```python
from build123d import *

# Parameters (mm, degrees)
F1_DEPTH = 63.5
F0_W     = 22.4716843884
F0_H     = 19.05
F2_DEPTH = 25.4
F3_DEPTH = 15.875
F5_R     = 6.35


# Not quite as in the source:
# - the program builds the solid bodies; features that only make, move or delete a surface that nothing else refers to are left out


with BuildPart() as f1:
    # F0 (on Front) → F1 (new body, symmetric)
    with BuildSketch(Plane.XZ):
        Polygon((22.225, 9.525), (-41.275, 9.525), (-41.275, -9.525), (41.275, -9.525), (41.275, 9.525), align=None)
    extrude(amount=F1_DEPTH, both=True)

    # F0 (on Front) → F2 (join, symmetric)
    with BuildSketch(Plane.XZ):
        with BuildLine():
            Line((22.225, 27.0002), (22.225, 9.525))
            Line((22.225, 9.525), (41.275, 9.525))
            Line((41.275, 9.525), (41.275, 27.0002))
            ThreePointArc((41.275, 27.0002), (45.9246798487, 38.2255201513), (57.15, 42.8752))
            Line((57.15, 42.8752), (60.325, 42.8752))
            Line((60.325, 42.8752), (60.325, 61.9252))
            Line((60.325, 61.9252), (57.15, 61.9252))
            ThreePointArc((57.15, 61.9252), (32.4542956671, 51.6959043329), (22.225, 27.0002))
        make_face()
        with Locations((71.5608421942, 52.4002)):
            Rectangle(F0_W, F0_H)
    extrude(amount=F2_DEPTH, both=True)

    # F0 (on Front) → F3 (join)
    with BuildSketch(Plane.XZ):
        with BuildLine():
            add(Edge.make_bspline(
                [(-41.275, 9.525), (-37.7052687109, 41.8739132583), (35.1902469993, 68.9807906747), (57.15, 61.9252)],
                knots=[0, 0, 0, 0, 111.5045361635, 111.5045361635, 111.5045361635, 111.5045361635], degree=3))
            Line((-41.275, 9.525), (22.225, 9.525))
            Line((22.225, 9.525), (22.225, 27.0002))
            ThreePointArc((22.225, 27.0002), (32.4542956671, 51.6959043329), (57.15, 61.9252))
        make_face()
    extrude(amount=F3_DEPTH)

    # F5
    f5_edges = [f1.edges().sort_by_distance(p)[0] for p in [
        (41.275, -63.5, 0),
        (-41.275, -63.5, 0),
        (-41.275, 63.5, 0),
        (41.275, 63.5, 0),
    ]]
    fillet(f5_edges, radius=F5_R)


solid = f1.part
```
Read the model definition and answer for the solid it produces. Units are mm, in the model's axes. A direction names the side the tool comes from. Round coordinates to 2 decimals unless told otherwise and drop trailing zeros. Write each loop counter-clockwise with the first axis right and the second up, starting at its lowest first coordinate (ties: lowest second). Pieces come first, ordered by that corner, then holes. Notation, with made-up numbers: (11.5, -29.75) - (53.5, -29.75) arc R18 cw to (53.5, -23.75) - close; hole circle Ø4 at (48, 53.5). An arc over 180 degrees is marked (long way). One line per item, written item: value.
Q1. Find section D-D (y = 35.5). Determine the outline of the cut face in (x, z) (3 decimals), and give its area (3 significant figures).
The answers:
outline: (-41.275, -9.525) - (41.275, -9.525) - (41.275, 9.525) - (-41.275, 9.525) - close
area: 1,570 mm2
Q2. Find section A-A (z = 2.5). Determine the outline of the cut face in (x, y) (3 decimals), and give its area (3 significant figures).
The answers:
outline: (-41.275, -57.15) arc R6.35 ccw to (-34.925, -63.5) - (34.925, -63.5) arc R6.35 ccw to (41.275, -57.15) - (41.275, 57.15) arc R6.35 ccw to (34.925, 63.5) - (-34.925, 63.5) arc R6.35 ccw to (-41.275, 57.15) - close
area: 10,400 mm2
Q3. Find section B-B (y = -19). Determine the outline of the cut face in (x, z) (3 decimals).
The answers:
outline: (-41.275, -9.525) - (41.275, -9.525) - (41.275, 27) arc R15.875 cw to (57.15, 42.875) - (82.797, 42.875) - (82.797, 61.925) - (57.15, 61.925) arc R34.925 ccw to (22.225, 27) - (22.225, 9.525) - (-41.275, 9.525) - close
Q4. Straight lines are drawn through the part: line 1 (Z direction, x = 4.5, y = 6) (3 decimals); line 2 (X direction, y = -19, z = -6) (3 decimals); line 3 (Y direction, x = -6.5, z = 10) (3 decimals). For each, find the intervals that lie inside material, in ascending order. Write a range as from..to.
The answers:
line 1: z = -9.525..9.525
line 2: x = -41.275..41.275
line 3: y = -15.875..0
Q5. Find section C-C (x = 64.5). Determine the outline of the cut face in (y, z), and give its area (3 significant figures).
The answers:
outline: (-25.4, 42.88) - (25.4, 42.88) - (25.4, 61.93) - (-25.4, 61.93) - close
area: 968 mm2
Q6. Each of these flat-tipped pins is pushed along its axis until it touches: P1, Ø1.5, axis at x = 14, z = 42.5, coming from the +Y side; P2, Ø7.5, axis at x = 67, y = -8.5, coming from the -Z side; P3, Ø1, axis at y = 3, z = 11.5, coming from the -X side (3 decimals); P4, Ø15.5, axis at x = 52, z = 29.5, coming from the +Y side. Where does it stop, or does it pass through?
The answers:
P1: stops at y = 0
P2: stops at z = 42.88
P3: stops at x = 22.225
P4: passes through
Q7. Which of the six approach directions +Z, -Z, +X, -X, +Y, -Y give full straight-line access (tool end or side, diameter ignored) to faces 1 (the flat face through (70, 0, 61.925)), 2 (the flat face through (22.225, -21, 18)), 3 (the flat face through (70, 0, 42.875))?
The answers:
face 1: +Z, +X, +Y, -Y
face 2: +Z, -X, -Y
face 3: -Z, +X, +Y, -Y
